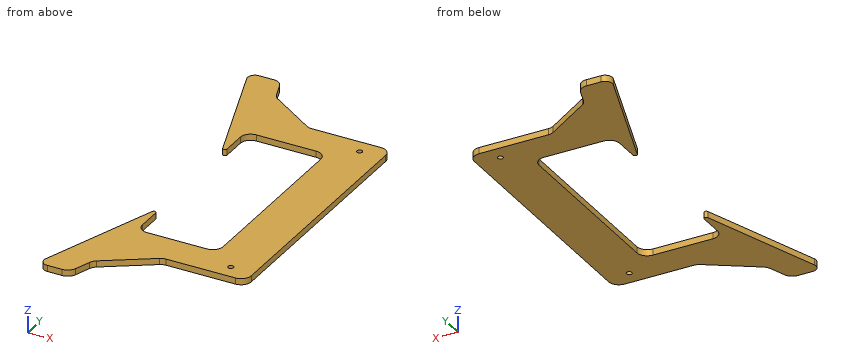
```python
from build123d import *

# Parameters (mm, degrees)
ESBO_O1_R                = 2.6
RESSALTO_EXTRUS_O1_DEPTH = 6
FILETE1_R                = 2
FILETE3_R                = 10
FILETE4_R                = 7


with BuildPart() as part:
    # Esboço1 → Ressalto-extrusão1 (new body)
    with BuildSketch(Plane.XY):
        Polygon((-100.5, 95.8), (-22.5, 95.8), (-22.5, -95.8), (-100.5, -95.8), (-100.5, -50.8), (-147.5, -185.8), (-116.203703704, -185.8), (-107.5, -160.8), (-57.5, -127.8), (22.5, -127.8), (22.5, 127.8), (-57.5, 127.8), (-107.5, 160.8), (-116.203703704, 185.8), (-147.5, 185.8), (-100.5, 50.8), align=None)
        with Locations((0, 113.2)):
            Circle(ESBO_O1_R, mode=Mode.SUBTRACT)
        with Locations((0, -113.2)):
            Circle(ESBO_O1_R, mode=Mode.SUBTRACT)
    extrude(amount=RESSALTO_EXTRUS_O1_DEPTH)

    # Filete1
    filete1_edges = [part.edges().sort_by_distance(p)[0] for p in [
        (-100.5, -50.8, 3),
        (-100.5, 50.8, 3),
    ]]
    fillet(filete1_edges, radius=FILETE1_R)

    # Filete3
    filete3_edges = [part.edges().sort_by_distance(p)[0] for p in [
        (-57.5, 127.8, 3),
        (22.5, 127.8, 3),
        (22.5, -127.8, 3),
        (-57.5, -127.8, 3),
        (-107.5, -160.8, 3),
        (-116.203703704, -185.8, 3),
        (-100.5, -95.8, 3),
        (-22.5, -95.8, 3),
        (-22.5, 95.8, 3),
        (-100.5, 95.8, 3),
        (-116.203703704, 185.8, 3),
        (-107.5, 160.8, 3),
    ]]
    fillet(filete3_edges, radius=FILETE3_R)

    # Filete4
    filete4_edges = [part.edges().sort_by_distance(p)[0] for p in [
        (-147.5, -185.8, 3),
        (-147.5, 185.8, 3),
    ]]
    fillet(filete4_edges, radius=FILETE4_R)


solid = part.part
```
The model under review builds one solid part; all positions refer to its coordinate system, in mm. Round coordinates to 2 decimals unless told otherwise and drop trailing zeros. Loops run counter-clockwise (first coordinate to the right, second up) from the corner with the lowest first, then second, coordinate; pieces in that order, holes last. Notation, with made-up numbers: (89, -6.5) - (122, -6.5) arc R26 cw to (122, 19.5) - close; hole circle Ø4 at (-2, -24.75). An arc over 180 degrees is marked (long way). Use a Markdown table: item, result. Add a question column.
Q1. Add section C-C (y = -67). State the section outline as (x, z) points.
Q2. Add section B-B (x = -74). State the section outline as (y, z) points, plus the area to 3 significant figures.
Q3. Add section D-D (x = -8). State the section outline as (y, z) points, plus the area to 3 significant figures.
Q4. For probe 1 along Y at (x, z) = (0, 3.85); probe 2 along Y at (x, z) = (-53, 4.5); probe 3 along X at (y, z) = (13.5, 3.45), list the stretches that pass through material, from the lowest coordinate up.
Q5. Insertion check: pin 1 Ø8.5 at (x, y) = (0, -113.2) entering from -Z; pin 2 Ø2 at (y, z) = (33, 5) entering from -X; pin 3 Ø1.8 at (x, z) = (-65, 4) entering from +Y; pin 4 Ø2 at (x, z) = (-2.5, 3) entering from +Y. Each pin has a flat end and moves straight along its axis. Give the tip position at first contact, or say it passes through.
Q6. Add section A-A (z = 1.15). State how many separate pieces and enclosed holes the cut face has, plus the area to 3 significant figures.
Worked answers:
| question | item | result |
|---|---|---|
| 1 | outline | (-106.14, 0) - (-100.5, 0) - (-100.5, 6) - (-106.14, 6) - close; (-22.5, 0) - (22.5, 0) - (22.5, 6) - (-22.5, 6) - close |
| 2 | outline | (-138.69, 0) - (-95.8, 0) - (-95.8, 6) - (-138.69, 6) - close; (95.8, 0) - (138.69, 0) - (138.69, 6) - (95.8, 6) - close |
| 2 | area | 515 mm² |
| 3 | outline | (-127.8, 0) - (127.8, 0) - (127.8, 6) - (-127.8, 6) - close |
| 3 | area | 1,530 mm² |
| 4 | probe 1 | -127.8 to -115.8, -110.6 to 110.6, 115.8 to 127.8 |
| 4 | probe 2 | -127.8 to -95.8, 95.8 to 127.8 |
| 4 | probe 3 | -22.5 to 22.5 |
| 5 | pin 1 | z = 0 |
| 5 | pin 2 | x = -22.5 |
| 5 | pin 3 | y = 133.34 |
| 5 | pin 4 | y = 127.8 |
| 6 | separate pieces | 1 |
| 6 | enclosed holes | 2 |
| 6 | area | 23,400 mm² |
